Could you check a few things on this model? Use its own coordinates, in mm. Face numbers are marked on the shaded views. Round coordinates to 2 decimals unless told otherwise and drop trailing zeros. Write each loop counter-clockwise with the first axis right and the second up, starting at its lowest first coordinate (ties: lowest second). Pieces come first, ordered by that corner, then holes. Notation, with made-up numbers: (-18, 25.5) -> (-8, 25.5) arc R17 ccw to (-8, 44.5) -> close; hole circle Ø4 at (66.5, 78.25). An arc over 180 degrees is marked (long way). Answer as CSV lines item,"result". Start each with the question number.
Q1. Will these pins go through, and if not, where does the flat tip stop? pin 1 Ø3 at (y, z) = (-8.5, -8.5) entering from -X; pin 2 Ø1 at (x, z) = (-1.5, -7) entering from +Y; pin 3 Ø13 at (x, y) = (0, 0) entering from -Z.
Q2. Imagine slicing it at A-A on y = 0. Please give me the cut outline in (x, z).
Q3. If I drill on line 1 (X direction, y = 0, z = -3); line 2 (Y direction, x = 0, z = -5); line 3 (X direction, y = 4.5, z = -8.5), over which ranges is the centre line in solid material (lowest first)? Write a range as [from, to].
Q4. Imagine slicing it at B-B on x = 0. Please give me the cut outline in (y, z).
Q5. If we mould it in two halves opening along X, with no side actions, what happens to the marked faces 1, 2 and 3? For each: pulls with the +X half, pulls with the -X half, needs draft (parallel to the pull), parting line crosses it, or undercut.
Q6. Imagine slicing it at C-C on z = 0. Please give me the cut outline in (x, y).
Q7. Imagine slicing it at D-D on x = 10.5. Please give me the cut outline in (y, z), and give its area (3 significant figures).
from build123d import *

# Parameters (mm, degrees)
F1_DEPTH      = 15
F1_DEPTH_BACK = 15
F3_R          = 2
F4_DEPTH      = 5.5
F5_R          = 2


with BuildPart() as f1:
    # F0 (on Top) → F1 (new body, two sides)
    with BuildSketch(Plane.XY) as f1_sk:
        with BuildLine():
            ThreePointArc((-8.801296, 8.371598), (-9.502154, 8.518054), (-10.121276, 8.158417))
            ThreePointArc((-10.121276, 8.158417), (-12.52886, -3.468091), (-4.485436, -12.201675))
            ThreePointArc((-4.485436, -12.201675), (-4.076574, -12.883522), (-3.349904, -12.560977))
            ThreePointArc((-3.349904, -12.560977), (-2.728421, -12.710457), (-2.100341, -12.829208))
            ThreePointArc((-2.100341, -12.829208), (-1.570219, -13.413333), (-0.919519, -12.967439))
            ThreePointArc((-0.919519, -12.967439), (0, -13), (0.919519, -12.967439))
            ThreePointArc((0.919519, -12.967439), (1.570219, -13.413333), (2.100341, -12.829208))
            ThreePointArc((2.100341, -12.829208), (2.728421, -12.710457), (3.349904, -12.560977))
            ThreePointArc((3.349904, -12.560977), (4.076574, -12.883522), (4.485436, -12.201675))
            ThreePointArc((4.485436, -12.201675), (12.52886, -3.468091), (10.121276, 8.158417))
            ThreePointArc((10.121276, 8.158417), (9.502154, 8.518054), (8.801296, 8.371598))
            Line((8.801296, 8.371598), (8.716739, 8.317146))
            ThreePointArc((8.716739, 8.317146), (8.270881, 7.635389), (8.480163, 6.848126))
            ThreePointArc((8.480163, 6.848126), (0, -10.9), (-8.480163, 6.848126))
            ThreePointArc((-8.480163, 6.848126), (-8.270881, 7.635389), (-8.716739, 8.317146))
            Line((-8.716739, 8.317146), (-8.801296, 8.371598))
        make_face()
    extrude(amount=F1_DEPTH)
    extrude(f1_sk.sketch, amount=-F1_DEPTH_BACK)

    # F3 (on offset) → F4 (join)
    with BuildSketch(Plane.XZ.offset(11.5)):
        Circle(F3_R)
    extrude(amount=-F4_DEPTH)

    # F5
    f5_edges = [f1.edges().sort_by_distance(p)[0] for p in [
        (-2, -6, 0),
    ]]
    fillet(f5_edges, radius=F5_R)


solid = f1.part
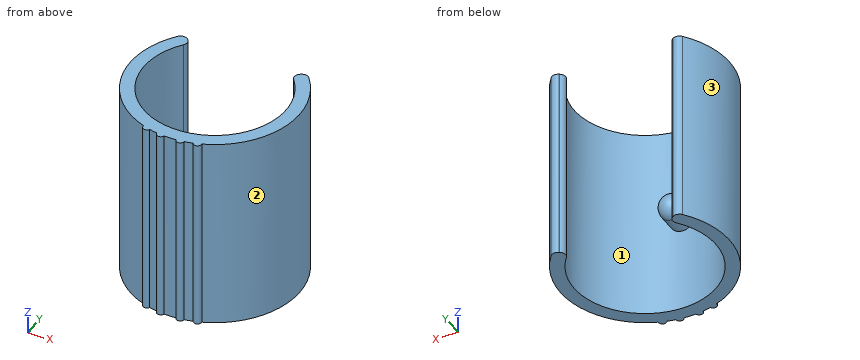
Checks:
1,pin 1,"x = -10.95"
1,pin 2,"y = -10.71"
1,pin 3,"z = -1.32"
2,outline,"(-13, -15) -> (-10.9, -15) -> (-10.9, 15) -> (-13, 15) -> close; (10.9, -15) -> (13, -15) -> (13, 15) -> (10.9, 15) -> close"
3,line 1,"[-13, -10.9], [10.9, 13]"
3,line 2,"[-13, -10.9]"
3,line 3,"[-12.2, -9.93], [9.93, 12.2]"
4,outline,"(-13, -15) -> (-10.9, -15) -> (-10.9, -2) -> (-8, -2) arc R2 ccw to (-8, 2) -> (-10.9, 2) -> (-10.9, 15) -> (-13, 15) -> close"
5,face 1,"undercut"
5,face 2,"pulls with the +X half"
5,face 3,"pulls with the -X half"
6,outline,"(-10.12, 8.16) arc R13 ccw to (-4.49, -12.2) arc R0.6 ccw to (-3.35, -12.56) arc R13 ccw to (-2.1, -12.83) arc R0.6 ccw to (-0.92, -12.97) arc R13 ccw to (0.92, -12.97) arc R0.6 ccw to (2.1, -12.83) arc R13 ccw to (3.35, -12.56) arc R0.6 ccw to (4.49, -12.2) arc R13 ccw to (10.12, 8.16) arc R1 ccw to (8.8, 8.37) -> (8.72, 8.32) arc R1 ccw to (8.48, 6.85) arc R10.9 cw to (2, -10.71) -> (2, -8) arc R2 ccw to (-2, -8) -> (-2, -10.71) arc R10.9 cw to (-8.48, 6.85) arc R1 ccw to (-8.72, 8.32) -> (-8.8, 8.37) arc R1 ccw to start"
7,outline,"(-7.66, -15) -> (-2.93, -15) -> (-2.93, 15) -> (-7.66, 15) -> close; (2.93, -15) -> (7.66, -15) -> (7.66, 15) -> (2.93, 15) -> close"
7,area,"284 mm^2"
